```python
from build123d import *

# Parameters (mm, degrees)
F0_W      = 203.2
F0_H      = 101.6
F1_DEPTH  = 12.7
F2_W      = 203.2
F2_H      = 6.35
F3_DEPTH  = 6.35
F5_DEPTH  = 6.35
F7_DEPTH  = 6.35
F8_W      = 25.4
F8_H      = 12.7
F9_DEPTH  = 1.5875
F10_R     = 1.5875
F11_DEPTH = 6.35
F12_R     = 1.5875
F13_DEPTH = 6.35


with BuildPart() as f1:
    # F0 (on Front) → F1 (new body)
    with BuildSketch(Plane.XZ):
        with Locations((3.333623, 0)):
            Rectangle(F0_W, F0_H)
    extrude(amount=F1_DEPTH)

    # F2 (on face) → F3 (cut)
    with BuildSketch(Plane(origin=(0, 0, 0), x_dir=(-1, 0, 0), z_dir=(0, 1, 0))):
        with Locations((-3.333623, -41.275)):
            Rectangle(F2_W, F2_H)
    extrude(amount=-F3_DEPTH, mode=Mode.SUBTRACT)

    # F4 (on face) → F5 (cut)
    with BuildSketch(Plane(origin=(-98.266377, 0, 0), x_dir=(0, -1, 0), z_dir=(-1, 0, 0))):
        with BuildLine():
            ThreePointArc((12.7, 19.05), (6.35, 25.4), (12.7, 31.75))
            Line((12.7, 31.75), (12.7, 50.8))
            Line((12.7, 50.8), (0, 50.8))
            Line((0, 50.8), (0, -38.1))
            Line((0, -38.1), (6.35, -38.1))
            Line((6.35, -38.1), (6.35, -44.45))
            Line((6.35, -44.45), (0, -44.45))
            Line((0, -44.45), (0, -50.8))
            Line((0, -50.8), (12.7, -50.8))
            Line((12.7, -50.8), (12.7, -31.75))
            ThreePointArc((12.7, -31.75), (6.35, -25.4), (12.7, -19.05))
            Line((12.7, -19.05), (12.7, -6.35))
            ThreePointArc((12.7, -6.35), (6.35, 0), (12.7, 6.35))
            Line((12.7, 6.35), (12.7, 19.05))
        make_face()
    extrude(amount=-F5_DEPTH, mode=Mode.SUBTRACT)

    # F6 (on face) → F7 (cut)
    with BuildSketch(Plane.YZ.offset(104.933623)):
        with BuildLine():
            ThreePointArc((-12.7, 31.75), (-6.35, 25.4), (-12.7, 19.05))
            Line((-12.7, 19.05), (-12.7, 6.35))
            ThreePointArc((-12.7, 6.35), (-6.35, 0), (-12.7, -6.35))
            Line((-12.7, -6.35), (-12.7, -19.05))
            ThreePointArc((-12.7, -19.05), (-6.35, -25.4), (-12.7, -31.75))
            Line((-12.7, -31.75), (-12.7, -50.8))
            Line((-12.7, -50.8), (0, -50.8))
            Line((0, -50.8), (0, -44.45))
            Line((0, -44.45), (-6.35, -44.45))
            Line((-6.35, -44.45), (-6.35, -38.1))
            Line((-6.35, -38.1), (0, -38.1))
            Line((0, -38.1), (0, 50.8))
            Line((0, 50.8), (-12.7, 50.8))
            Line((-12.7, 50.8), (-12.7, 31.75))
        make_face()
    extrude(amount=-F7_DEPTH, mode=Mode.SUBTRACT)

    # F8 (on face) → F9 (cut)
    with BuildSketch(Plane.XY.offset(50.8)):
        with Locations((-53.816377, -6.35)):
            Rectangle(F8_W, F8_H)
        with Locations((60.483623, -6.35)):
            Rectangle(F8_W, F8_H)
    extrude(amount=-F9_DEPTH, mode=Mode.SUBTRACT)

    # F10 (on face) → F11 (cut)
    with BuildSketch(Plane.XY.offset(49.2125)):
        with Locations((-60.166377, -6.35)):
            Circle(F10_R)
        with Locations((-47.466377, -6.35)):
            Circle(F10_R)
    extrude(amount=-F11_DEPTH, mode=Mode.SUBTRACT)

    # F12 (on face) → F13 (cut)
    with BuildSketch(Plane.XY.offset(49.2125)):
        with Locations((54.133623, -6.35)):
            Circle(F12_R)
        with Locations((66.833623, -6.35)):
            Circle(F12_R)
    extrude(amount=-F13_DEPTH, mode=Mode.SUBTRACT)


solid = f1.part
```
CAD build for the part. Positions are in the model's coordinates, mm. A direction names the side the tool comes from. Round coordinates to 2 decimals unless told otherwise and drop trailing zeros. Write each loop counter-clockwise with the first axis right and the second up, starting at its lowest first coordinate (ties: lowest second). Pieces come first, ordered by that corner, then holes. Notation, with made-up numbers: (19.5, 40) - (72.5, 40) arc R29 cw to (72.5, 78) - close; hole circle Ø8 at (31.5, 4). An arc over 180 degrees is marked (long way). Return JSON: item names as keys, results as strings. Group by question number.
Item 1: Band-saw the part on A-A on z = 25.4. List the corners of the cut face in (x, y).
Item 2: Flat gauge pins, fed straight in: pin 1 Ø1 at (x, y) = (-44.5, -2) entering from +Z; pin 2 Ø1.3 at (y, z) = (-3.5, 50) entering from -X; pin 3 Ø1.9 at (x, y) = (54.13, -6.35) entering from +Z; pin 4 Ø4 at (y, z) = (-6.5, -2.5) entering from +X. Where does each tip first touch, or does it go through?
Item 3: Mould opens along X. For faces 4 (the face through (104.934, -10, 0)), 5 (the face through (60, -6, 49.212)), 6 (the face through (-95.14, -6.35, 25.26)) say: +X half, -X half, draft (parallel to the pull), parting line (faces both ways), or undercut.
Item 4: 3-axis set-ups, long thin cutter, end or side, ignore diameter. For faces 1 (the face through (101.8, -6.35, 25.54)), 2 (the face through (5, -6.35, -41)), 3 (the face through (-95.14, -6.35, -0.14)): which of +Z, -Z, +X, -X, +Y, -Y reach the whole face in a straight line?
Item 5: Band-saw the part on C-C on z = 11.5. List the corners of the cut face in (x, y).
Item 6: Band-saw the part on B-B on x = -77.5. List the corners of the cut face in (y, z), plus the area to 3 significant figures.
Item 7: Probe probe 1 along Z at (x, y) = (-4, -4.25); probe 2 along Z at (x, y) = (60, -1); probe 3 along X at (y, z) = (-5, -5). List the from-to ranges inside material, lowest first.
Resolved:
{
 "1": {"outline": "(-98.27, -12.7) - (104.93, -12.7) - (104.93, -6.35) - (98.58, -6.35) - (98.58, 0) - (-91.92, 0) - (-91.92, -6.35) - (-98.27, -6.35) - close"},
 "2": {"pin 1": "stops at z = 49.21", "pin 2": "stops at x = -91.92", "pin 3": "stops at z = 42.86", "pin 4": "stops at x = 104.93"},
 "3": {"face 4": "+X half", "face 5": "undercut", "face 6": "draft"},
 "4": {"face 1": "+X, +Y", "face 2": "+X, -X, +Y", "face 3": "-X, +Y"},
 "5": {"outline": "(-91.92, -12.7) - (98.58, -12.7) - (98.58, 0) - (-91.92, 0) - close"},
 "6": {"outline": "(-12.7, -50.8) - (0, -50.8) - (0, -44.45) - (-6.35, -44.45) - (-6.35, -38.1) - (0, -38.1) - (0, 50.8) - (-12.7, 50.8) - close", "area": "1,250 mm²"},
 "7": {"probe 1": "z = -50.8 to -44.45, -38.1 to 50.8", "probe 2": "z = -50.8 to -44.45, -38.1 to 49.21", "probe 3": "x = -91.92 to 98.58"}
}
